from build123d import *

# Parameters (mm, degrees)
SKETCH1_W           = 70
SKETCH1_H           = 45
BOSS_EXTRUDE1_DEPTH = 35
SKETCH2_R           = 25.5
BOSS_EXTRUDE2_DEPTH = 90
SKETCH3_R           = 3
CUT_EXTRUDE1_DEPTH  = 10


with BuildPart() as part:
    # Sketch1 → Boss-Extrude1 (new body)
    with BuildSketch(Plane.XY):
        Rectangle(SKETCH1_W, SKETCH1_H)
    extrude(amount=BOSS_EXTRUDE1_DEPTH)

    # Sketch2 → Boss-Extrude2 (add)
    with BuildSketch(Plane.XY.offset(35)):
        Circle(SKETCH2_R)
    extrude(amount=BOSS_EXTRUDE2_DEPTH)

    # Sketch3 → Cut-Extrude1 (cut)
    with BuildSketch(Plane(origin=(0, 22.5, 0), x_dir=(1, 0, 0), z_dir=(0, 1, 0))):
        with Locations((0, -17.5)):
            Circle(SKETCH3_R)
    extrude(amount=-CUT_EXTRUDE1_DEPTH, mode=Mode.SUBTRACT)


solid = part.part
Here's how the part is built. I have some questions about the finished solid (model axes, mm). A direction names the side the tool comes from. Round coordinates to 2 decimals unless told otherwise and drop trailing zeros. Order: outer loops, then holes, each group sorted by start corner. A loop starts at its lowest first (then second) coordinate and runs counter-clockwise, first axis right, second up. Notation, with made-up numbers: (48, 57.5) -> (91, 57.5) arc R23 cw to (91, 72.5) -> close; hole circle Ø6 at (78, -22). An arc over 180 degrees is marked (long way). Return JSON: item names as keys, results as strings.
Q1. If we section it at A-A on x = 0: List the corners of the cut face in (y, z) for me, plus the area to 4 significant figures.
Filled sheet:
{"outline": "(-25.5, 35) -> (-22.5, 35) -> (-22.5, 0) -> (22.5, 0) -> (22.5, 14.5) -> (12.5, 14.5) -> (12.5, 20.5) -> (22.5, 20.5) -> (22.5, 35) -> (25.5, 35) -> (25.5, 125) -> (-25.5, 125) -> close", "area": "6,105 mm^2"}
Q2. If we section it at D-D on z = 89.5: List the corners of the cut face in (x, y) for me, plus the area to 3 significant figures.
Filled sheet:
{"outline": "circle Ø51 at (0, 0)", "area": "2,040 mm^2"}
Q3. If we section it at B-B on z = 17.5: List the corners of the cut face in (x, y) for me.
Filled sheet:
{"outline": "(-35, -22.5) -> (35, -22.5) -> (35, 22.5) -> (3, 22.5) -> (3, 12.5) -> (-3, 12.5) -> (-3, 22.5) -> (-35, 22.5) -> close"}
Q4. For pin 1 Ø1 at (x, z) = (8, 23) entering from -Y; pin 2 Ø3 at (x, z) = (-0.5, 17) entering from +Y; pin 3 Ø6 at (x, z) = (18, 110.5) entering from -Y, each with a flat end and sliding along its axis, tell me the tip position at first contact or that it passes through.
Filled sheet:
{"pin 1": "stops at y = -22.5", "pin 2": "stops at y = 12.5", "pin 3": "stops at y = -20.62"}
Q5. Which directions (+Z, -Z, +X, -X, +Y, -Y) give clear straight access to the entire face, cutting with the end or side of a thin tool? Please do faces 5 (the flat face through (0, 22.5, 21)), 6 (the flat face through (0, 0, 125)), 7 (the flat face through (0, -22.5, 17)), 8 (the flat face through (-29, 0, 35)), 9 (the cylindrical face through (-5.5, -24.9, 79.4)).
Filled sheet:
{"face 5": "-Z, +X, -X, +Y", "face 6": "+Z, +X, -X, +Y, -Y", "face 7": "-Z, +X, -X, -Y", "face 8": "+Z, -X", "face 9": "+Z"}
Q6. I need wall thicknesses on line 1 along Z through (x, y) = (0, 19); line 2 along X through (y, z) = (15, 17.5); line 3 along Y through (x, z) = (-23, 9). Which ranges of each line are inside material? Lowest first, please. Write a range as from..to.
Filled sheet:
{"line 1": "z = 0..14.5, 20.5..125", "line 2": "x = -35..-3, 3..35", "line 3": "y = -22.5..22.5"}
Q7. If we mould it in two halves opening along X, with no side actions, what happens to faces 1 (the flat face through (-35, 0, 17)), 2 (the cylindrical face through (-0.65, 17.57, 20.43)), 3 (the flat face through (0, 12.5, 17)), 4 (the flat face through (0, 0, 0))? For each: released by +X, released by -X, zero draft, split by the parting line, or undercut.
Filled sheet:
{"face 1": "released by -X", "face 2": "undercut", "face 3": "undercut", "face 4": "zero draft"}
Q8. If we section it at C-C on y = 0: List the corners of the cut face in (x, z) for me.
Filled sheet:
{"outline": "(-35, 0) -> (35, 0) -> (35, 35) -> (25.5, 35) -> (25.5, 125) -> (-25.5, 125) -> (-25.5, 35) -> (-35, 35) -> close"}
